from build123d import *

# Parameters (mm, degrees)
SKETCH_1_R      = 1.5
EXTRUDE_1_DEPTH = 3


with BuildPart() as part:
    # 草圖1 → 填料-伸長1 (new body)
    with BuildSketch(Plane.XY):
        with BuildLine():
            Line((58.3003, 1), (142.0003, 1))
            ThreePointArc((142.0003, 1), (149.071310355, 3.928960355), (152.0002, 11))
            Line((152.0002, 11), (152.0002, 86))
            ThreePointArc((152.0002, 86), (149.071335355, 93.071064644), (142.0003, 96))
            Line((142.0003, 96), (58.3003, 96))
            ThreePointArc((58.3003, 96), (51.584341425, 93.406620638), (48.3003, 87))
            Line((48.3003, 87), (48.3003, 11))
            ThreePointArc((48.3003, 11), (51.22925, 3.92895), (58.3003, 1))
        make_face()
        with Locations((73.150306055, 21.499982809)):
            Circle(SKETCH_1_R, mode=Mode.SUBTRACT)
        with Locations((58.3003, 11)):
            Circle(SKETCH_1_R, mode=Mode.SUBTRACT)
        with Locations((142.000224541, 10.999975458)):
            Circle(SKETCH_1_R, mode=Mode.SUBTRACT)
        with Locations((127.150308327, 21.499982809)):
            Circle(SKETCH_1_R, mode=Mode.SUBTRACT)
        with Locations((142.000224541, 86)):
            Circle(SKETCH_1_R, mode=Mode.SUBTRACT)
        with Locations((127.150308327, 75.500030546)):
            Circle(SKETCH_1_R, mode=Mode.SUBTRACT)
        with Locations((73.150306055, 75.500030546)):
            Circle(SKETCH_1_R, mode=Mode.SUBTRACT)
        with Locations((58.342751992, 86)):
            Circle(SKETCH_1_R, mode=Mode.SUBTRACT)
        with BuildLine():
            Line((124.449289873, 24.90807964), (143.091425497, 43.550215264))
            ThreePointArc((143.091425497, 43.550215264), (145.141678029, 48.499962732), (143.091425497, 53.4497102))
            Line((143.091425497, 53.4497102), (105.100047468, 91.441088229))
            ThreePointArc((105.100047468, 91.441088229), (100.1503, 93.491340761), (95.200552532, 91.441088229))
            Line((95.200552532, 91.441088229), (76.558416908, 72.798952605))
            Line((76.558416908, 72.798952605), (57.209174503, 53.4497102))
            ThreePointArc((57.209174503, 53.4497102), (55.158921971, 48.499962732), (57.209174503, 43.550215264))
            Line((57.209174503, 43.550215264), (95.200552532, 5.558837235))
            ThreePointArc((95.200552532, 5.558837235), (100.1503, 3.508584704), (105.100047468, 5.558837235))
            Line((105.100047468, 5.558837235), (124.449289873, 24.90807964))
        make_face(mode=Mode.SUBTRACT)
    extrude(amount=EXTRUDE_1_DEPTH)


solid = part.part
Verification items for the finished model (mm, model axes). A direction names the side the tool comes from. Coordinates: 2 decimals unless noted, no trailing zeros. Order: outer loops, then holes, each group sorted by start corner. A loop starts at its lowest first (then second) coordinate and runs counter-clockwise, first axis right, second up. Notation, with made-up numbers: M 19.5,41 L 40.5,41 A8 ccw 40.5,54 Z; hole C 19,69.25 d10. An arc over 180 degrees is marked long. Return JSON: item names as keys, results as strings.
1) Access from +Z, -Z, +X, -X, +Y, -Y to the whole of each face (thin tool, end or side, straight path). Record for faces 5 (the flat face through (75.94, 24.82, 1.48)), 6 (the cylindrical face through (149.15, 92.99, 1.48)).
Answer list:
{"face 5": "+Z, -Z", "face 6": "+Z, -Z, +X, +Y"}
2) Cross-section at C-C, the plane z = 2.45. Count the separate pieces of the cut face and the enclosed holes in it, and give its area (3 significant figures).
Answer list:
{"separate pieces": "1", "enclosed holes": "9", "area": "5,160 mm2"}
3) Gauge pin test, flat end, axial feed: pin 1 (2.5 mm diameter, centred on x = 73.15, y = 75.5, fed in from -Z). Record the tip position at first contact, or that the pin passes through.
Answer list:
{"pin 1": "through"}
4) Cross-section at A-A, the plane y = 47. Record the boundary of the cut face in (x, z), and give its area (3 significant figures).
Answer list:
{"outline": "M 48.3,0 L 55.32,0 L 55.32,3 L 48.3,3 Z; M 144.98,0 L 152,0 L 152,3 L 144.98,3 Z", "area": "42.1 mm2"}
5) Cross-section at B-B, the plane x = 100.5. Record the boundary of the cut face in (y, z).
Answer list:
{"outline": "M 1,0 L 3.52,0 L 3.52,3 L 1,3 Z; M 93.48,0 L 96,0 L 96,3 L 93.48,3 Z"}
6) Release check for a two-part mould opening along Y. For faces 1 (the cylindrical face through (125.65, 75.57, 1.48)), 2 (the cylindrical face through (51.15, 4.01, 1.48)), 3 (the flat face through (101, 96, 1)), 4 (the flat face through (152, 48, 1)) record: +Y half, -Y half, draft (parallel to the pull), parting line (faces both ways), or undercut.
Answer list:
{"face 1": "undercut", "face 2": "-Y half", "face 3": "+Y half", "face 4": "draft"}
7) Thickness scan on L1, parallel to X at y = 86, z = 1.65; L2, parallel to Y at x = 100, z = 2.2; L3, parallel to X at y = 8.5, z = 2.6. Record the ranges inside material, lowest first. Write a range as [from, to].
Answer list:
{"L1": "[48.3, 56.84], [59.84, 89.76], [110.54, 140.5], [143.5, 152]", "L2": "[1, 3.51], [93.49, 96]", "L3": "[48.62, 92.26], [108.04, 151.68]"}
